```python
from build123d import *

# Parameters (mm, degrees)
F0_R     = 15.920661
F1_DEPTH = 25.4
F2_DEPTH = 25.4
F3_DEPTH = 50.8


with BuildPart() as f1:
    # F0 (on Top) → F1 (new body)
    with BuildSketch(Plane.XY):
        with BuildLine():
            ThreePointArc((-46.308367, -28.973528), (-17.604609, 0), (-46.308367, 28.973528))
            ThreePointArc((-46.308367, 28.973528), (-75.554202, 0), (-46.308367, -28.973528))
        make_face()
        with Locations((-46.579406, 0)):
            Circle(F0_R, mode=Mode.SUBTRACT)
    extrude(amount=F1_DEPTH)

    # F0 (on Top) → F2 (join)
    with BuildSketch(Plane.XY):
        with BuildLine():
            Line((46.842293, 28.102132), (-46.308367, 28.973528))
            ThreePointArc((-46.308367, 28.973528), (-17.604609, 0), (-46.308367, -28.973528))
            Line((-46.308367, -28.973528), (46.842293, -28.102132))
            ThreePointArc((46.842293, -28.102132), (74.682768, 0), (46.842293, 28.102132))
        make_face()
        with Locations((46.579406, 0)):
            Circle(F0_R, mode=Mode.SUBTRACT)
    extrude(amount=F2_DEPTH)

    # F0 (on Top) → F3 (join)
    with BuildSketch(Plane.XY):
        with BuildLine():
            ThreePointArc((-46.308367, -28.973528), (-17.604609, 0), (-46.308367, 28.973528))
            ThreePointArc((-46.308367, 28.973528), (-75.554202, 0), (-46.308367, -28.973528))
        make_face()
        with Locations((-46.579406, 0)):
            Circle(F0_R, mode=Mode.SUBTRACT)
    extrude(amount=F3_DEPTH)


solid = f1.part
```
Geometry: final body of the model. Coordinates: model frame, mm. Coordinates: 2 decimals unless noted, no trailing zeros. Write each loop counter-clockwise with the first axis right and the second up, starting at its lowest first coordinate (ties: lowest second). Pieces come first, ordered by that corner, then holes. Notation, with made-up numbers: M -18.75,40 L -0.75,40 A16 ccw -0.75,63 Z; hole C -13.5,53.5 d5. An arc over 180 degrees is marked long. Use CSV: the item, a comma, the result in double quotes. Start each with the question number.
1. Cut plane B-B on y = 0. Return the cut outline in (x, z).
2. Cut plane D-D on x = 51. Return the cut outline in (y, z), plus the area to 3 significant figures.
3. Cut plane A-A on z = 15. Return the cut outline in (x, y).
4. First-contact query: P1, Ø5, axis at x = 49, z = 7, coming from the +Y side; P2, Ø10, axis at y = -11.5, z = 6, coming from the +X side; P3, Ø1.5, axis at y = -6, z = 25, coming from the -X side; P4, Ø3, axis at x = 20.5, z = 27, coming from the -Y side. Flat tips, straight axial feed; report the tip coordinate or a pass-through.
5. Cut plane C-C on x = -25. Return the cut outline in (y, z), plus the area to 3 significant figures.
6. Ray query, probe 1 along X at (y, z) = (2, 14.5); probe 2 along Z at (x, y) = (32, -23.5); probe 3 along X at (y, z) = (-4, 41.5). Return the intervals inside material, ascending.
7. Mould query, pull axis X, two halves, no side actions, for faces 1 (the face through (13, 0, 25.4)), 2 (the face through (-59.21, -9.69, 25.04)), 3 (the face through (74.676, -0.614, 12.522)). Classes: pulls with the +X half, pulls with the -X half, needs draft (parallel to the pull), parting line crosses it, or undercut.
Entries:
1,outline,"M -75.55,0 L -62.5,0 L -62.5,50.8 L -75.55,50.8 Z; M -30.66,0 L 30.66,0 L 30.66,25.4 L -17.6,25.4 L -17.6,50.8 L -30.66,50.8 Z; M 62.5,0 L 74.68,0 L 74.68,25.4 L 62.5,25.4 Z"
2,outline,"M -27.75,0 L -15.29,0 L -15.29,25.4 L -27.75,25.4 Z; M 15.29,0 L 27.75,0 L 27.75,25.4 L 15.29,25.4 Z"
2,area,"633 mm²"
3,outline,"M -46.31,-28.97 L 46.84,-28.1 A28.1 ccw 46.84,28.1 L -46.31,28.97 A28.97 ccw long Z; hole C -46.58,0 d31.84; hole C 46.58,0 d31.84"
4,P1,"y = 28.11"
4,P2,"x = 73.92"
4,P3,"x = -75.07"
4,P4,"through"
5,outline,"M -28.77,0 L 28.77,0 L 28.77,25.4 L 19.34,25.4 L 19.34,50.8 L -19.34,50.8 L -19.34,25.4 L -28.77,25.4 Z"
5,area,"2,440 mm²"
6,probe 1,"-75.49 to -62.37, -30.78 to 30.78, 62.37 to 74.61"
6,probe 2,"0 to 25.4"
6,probe 3,"-75.28 to -61.99, -31.17 to -17.88"
7,face 1,"needs draft"
7,face 2,"undercut"
7,face 3,"pulls with the +X half"
